Geometry check sheet. Reference: the model listing, model coordinates, mm. Face numbers are marked on the shaded views. Give positions to 0.01 mm unless a question says otherwise; leave off trailing zeros. Order: outer loops, then holes, each group sorted by start corner. A loop starts at its lowest first (then second) coordinate and runs counter-clockwise, first axis right, second up.
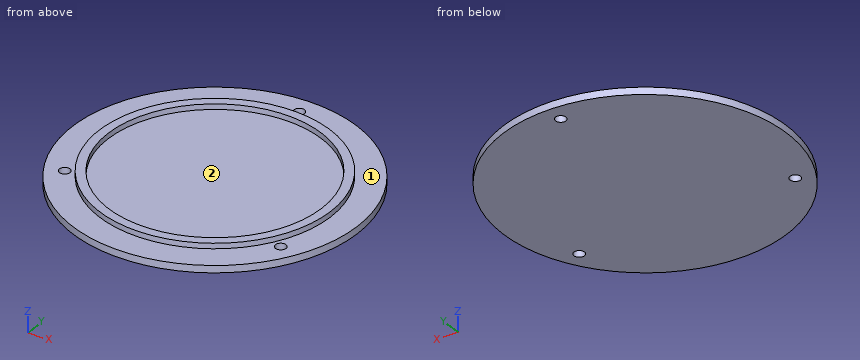
from build123d import *

# Parameters (mm, degrees)
SKETCH1_R           = 80
BOSS_EXTRUDE1_DEPTH = 4
SKETCH2_R           = 65
SKETCH2_R_2         = 60
BOSS_EXTRUDE2_DEPTH = 3
SKETCH3_R           = 3
CUT_EXTRUDE2_DEPTH  = 8


with BuildPart() as part:
    # Sketch1 → Boss-Extrude1 (new body)
    with BuildSketch(Plane.XY):
        Circle(SKETCH1_R)
    extrude(amount=BOSS_EXTRUDE1_DEPTH)

    # Sketch2 → Boss-Extrude2 (add)
    with BuildSketch(Plane.XY.offset(4)):
        Circle(SKETCH2_R)
        Circle(SKETCH2_R_2, mode=Mode.SUBTRACT)
    extrude(amount=BOSS_EXTRUDE2_DEPTH)

    # Sketch3 → Cut-Extrude2 (cut, through all)
    with BuildSketch(Plane(origin=(0, 0, 0), x_dir=(-1, 0, 0), z_dir=(0, 0, -1))):
        with Locations((0, 70)):
            Circle(SKETCH3_R)
        with Locations((60.621778265, -35)):
            Circle(SKETCH3_R)
        with Locations((-60.621778265, -35)):
            Circle(SKETCH3_R)
    extrude(amount=-CUT_EXTRUDE2_DEPTH, mode=Mode.SUBTRACT)


solid = part.part
Item 1: Sectioned sample at D-D (x = 40). Enter the section's corners in (y, z), and give its area (3 significant figures).
Reported:
outline: (-69.28, 0) - (69.28, 0) - (69.28, 4) - (51.23, 4) - (51.23, 7) - (44.72, 7) - (44.72, 4) - (-44.72, 4) - (-44.72, 7) - (-51.23, 7) - (-51.23, 4) - (-69.28, 4) - close
area: 593 mm2
Item 2: Draft check along X on the marked faces 1 and 2. Enter one of: released by +X, released by -X, zero draft, split by the parting line, or undercut.
Reported:
face 1: zero draft
face 2: undercut
Item 3: Gauge pin test, flat ends, axial feed: pin 1 (3.5 mm diameter, centred on x = -60.62, y = -35, fed in from +Z); pin 2 (9.5 mm diameter, centred on x = 60.62, y = -35, fed in from +Z); pin 3 (1.5 mm diameter, centred on x = 56, z = 5.5, fed in from +Y); pin 4 (2 mm diameter, centred on x = 56.5, z = 4, fed in from -Y). Record the tip position at first contact, or that the pin passes through.
Reported:
pin 1: passes through
pin 2: stops at z = 4
pin 3: stops at y = 34.24
pin 4: stops at y = -57.62
Item 4: Sectioned sample at C-C (y = 70). Enter the section's corners in (x, z).
Reported:
outline: (-38.73, 0) - (-3, 0) - (-3, 4) - (-38.73, 4) - close; (3, 0) - (38.73, 0) - (38.73, 4) - (3, 4) - close
Item 5: Sectioned sample at A-A (x = 0). Enter the section's corners in (y, z).
Reported:
outline: (-80, 0) - (67, 0) - (67, 4) - (65, 4) - (65, 7) - (60, 7) - (60, 4) - (-60, 4) - (-60, 7) - (-65, 7) - (-65, 4) - (-80, 4) - close; (73, 0) - (80, 0) - (80, 4) - (73, 4) - close
Item 6: Scan lines: L1, parallel to Y at x = 0, z = 1.9; L2, parallel to Z at x = 33, y = 48.5; L3, parallel to Y at x = 31, z = 5.5. Record each from-to range of solid material in increasing order.
Reported:
L1: y = -80 to 67, 73 to 80
L2: z = 0 to 4
L3: y = -57.13 to -51.37, 51.37 to 57.13
Item 7: Sectioned sample at B-B (y = 0). Enter the section's corners in (x, z).
Reported:
outline: (-80, 0) - (80, 0) - (80, 4) - (65, 4) - (65, 7) - (60, 7) - (60, 4) - (-60, 4) - (-60, 7) - (-65, 7) - (-65, 4) - (-80, 4) - close
